from build123d import *

# Parameters (mm, degrees)
F1_DEPTH  = 35
F0_R      = 7.6
F2_DEPTH  = 35
F3_R      = 2.15
F4_DEPTH  = 35.001
F5_R      = 3.65
F5_R_2    = 2.15
F6_DEPTH  = 31
F8_DEPTH  = 20.601
F9_W      = 0.5
F9_H      = 2
F10_DEPTH = 35.0010001
F11_R     = 1.45
F12_DEPTH = 13.851


with BuildPart() as f1:
    # F0 (on Top) → F1 (new body)
    with BuildSketch(Plane.XY):
        with BuildLine():
            ThreePointArc((10, -3.5156791662), (0, -10.6), (-10, -3.5156791662))
            Line((-10, -3.5156791662), (-10, -80.6))
            Line((-10, -80.6), (10, -80.6))
            Line((10, -80.6), (10, -3.5156791662))
        make_face()
    extrude(amount=-F1_DEPTH)

    # F0 (on Top) → F2 (join)
    with BuildSketch(Plane.XY):
        with BuildLine():
            Line((-3.25, 16.6), (-3.25, 10.0894747138))
            ThreePointArc((-3.25, 10.0894747138), (-9.4955609642, 4.7110850104), (-10, -3.5156791662))
            ThreePointArc((-10, -3.5156791662), (0, -10.6), (10, -3.5156791662))
            ThreePointArc((10, -3.5156791662), (9.4955609642, 4.7110850104), (3.25, 10.0894747138))
            Line((3.25, 10.0894747138), (3.25, 16.6))
            Line((3.25, 16.6), (-3.25, 16.6))
        make_face()
        Circle(F0_R, mode=Mode.SUBTRACT)
    extrude(amount=-F2_DEPTH)

    # F3 (on face) → F4 (cut, through all)
    with BuildSketch(Plane.XY):
        with Locations((0, -50.6)):
            Circle(F3_R)
        with Locations((0, -70.6)):
            Circle(F3_R)
    extrude(amount=-F4_DEPTH, mode=Mode.SUBTRACT)

    # F5 (on face) → F6 (cut)
    with BuildSketch(Plane(origin=(0, 0, -35), x_dir=(1, 0, 0), z_dir=(0, 0, -1))):
        with Locations((0, 70.6)):
            Circle(F5_R)
        with Locations((0, 70.6)):
            Circle(F5_R_2, mode=Mode.SUBTRACT)
        with Locations((0, 50.6)):
            Circle(F5_R)
        with Locations((0, 50.6)):
            Circle(F5_R_2, mode=Mode.SUBTRACT)
    extrude(amount=-F6_DEPTH, mode=Mode.SUBTRACT)

    # F7 (on face) → F8 (cut, through all)
    with BuildSketch(Plane.YZ.offset(10)):
        with BuildLine():
            Line((-80.6, -35), (-10.0156791662, -35))
            add(Edge.make_bspline(
                [(-10.0156791662, -35), (-10.0156791662, -5), (-80.6, -5)],
                knots=[0, 0, 0, 1.5707963268, 1.5707963268, 1.5707963268], degree=2, weights=[1, 0.7071067812, 1]))
            Line((-80.6, -5), (-80.6, -35))
        make_face()
    extrude(amount=-F8_DEPTH, mode=Mode.SUBTRACT)

    # F9 (on face) → F10 (cut, through all)
    with BuildSketch(Plane.XY):
        with BuildLine():
            Line((0.5, 16.6), (0, 16.6))
            Line((0, 16.6), (0, 7.6))
            ThreePointArc((0, 7.6), (0.2501355147, 7.5958825836), (0.5, 7.5835347959))
            Line((0.5, 7.5835347959), (0.5, 16.6))
        make_face()
        with BuildLine():
            Line((0, 0), (0, 7.6))
            ThreePointArc((0, 7.6), (-0.2501355147, 7.5958825836), (-0.5, 7.5835347959))
            Line((-0.5, 7.5835347959), (-0.5, 0))
            Line((-0.5, 0), (0, 0))
        make_face()
        with Locations((-0.25, 17.6)):
            Rectangle(F9_W, F9_H)
        with Locations((0.25, 17.6)):
            Rectangle(F9_W, F9_H)
        with BuildLine():
            ThreePointArc((0.5, 7.5835347959), (0.2501355147, 7.5958825836), (0, 7.6))
            Line((0, 7.6), (0, 0))
            Line((0, 0), (0.5, 0))
            Line((0.5, 0), (0.5, 7.5835347959))
        make_face()
        with BuildLine():
            Line((0, 7.6), (0, 16.6))
            Line((0, 16.6), (-0.5, 16.6))
            Line((-0.5, 16.6), (-0.5, 7.5835347959))
            ThreePointArc((-0.5, 7.5835347959), (-0.2501355147, 7.5958825836), (0, 7.6))
        make_face()
    extrude(amount=-F10_DEPTH, mode=Mode.SUBTRACT)

    # F11 (on face) → F12 (cut, through all)
    with BuildSketch(Plane.YZ.offset(3.25)):
        with Locations((13.6, -8.75)):
            Circle(F11_R)
        with Locations((13.6, -26.25)):
            Circle(F11_R)
    extrude(amount=-F12_DEPTH, mode=Mode.SUBTRACT)


solid = f1.part
Here's how the part is built. I have some questions about the finished solid (model axes, mm). A direction names the side the tool comes from. Give positions to 0.01 mm unless a question says otherwise; leave off trailing zeros. Write each loop counter-clockwise with the first axis right and the second up, starting at its lowest first coordinate (ties: lowest second). Pieces come first, ordered by that corner, then holes. Notation, with made-up numbers: (64.25, 84) -> (69.25, 84) arc R15 ccw to (69.25, 111) -> close; hole circle Ø10 at (87, 45.25). An arc over 180 degrees is marked (long way). Use one line per item in the form item = value. Start each with the question number.
1. If I drill on L1, parallel to Y at x = 0, z = -2.1; L2, parallel to Z at x = -2, y = 13.6; L3, parallel to X at y = -70.6, z = -2.1, over which ranges is the centre line in solid material (lowest first)?
2. Thinking about a two-plate mould opening in Y: for faces 1 (the face through (-0.791, -47.037, -5.832)), 2 (the face through (-10, -24, -9)), 3 (the face through (2, 16.6, -17)), which applies, +Y half, -Y half, draft (parallel to the pull), parting line (faces both ways), or undercut?
3. Imagine slicing it at A-A on y = 13.6. List the corners of the cut face in (x, z) for me.
4. Imagine slicing it at B-B on z = -26.25. State how many separate pieces and enclosed holes the cut face has, plus the area to 3 significant figures.
5. Will these pins go through, and if not, where does the flat tip stop? pin 1 Ø4 at (y, z) = (13.6, -26.25) entering from +X; pin 2 Ø3 at (x, y) = (5, -52) entering from -Z; pin 3 Ø2 at (y, z) = (-1, -24) entering from -X; pin 4 Ø1.5 at (x, z) = (-3, -26.5) entering from -Y.
6. On a 3-axis mill with a long thin cutter (end or side, diameter ignored), from which of +Z, -Z, +X, -X, +Y, -Y can I reach the whole of each face in a straight line? I mean faces 4 (the face through (10, -25, -9)), 5 (the face through (2, -69, -4)), 6 (the face through (3.25, 13, -17)). Say none if no direction works.
Entries:
q1.L1 = -80.6 to -72.75, -68.45 to -52.75, -48.45 to -7.6
q1.L2 = -35 to -27.7, -24.8 to -10.2, -7.3 to 0
q1.L3 = -10 to -2.15, 2.15 to 10
q2.face_1 = undercut
q2.face_2 = draft
q2.face_3 = +Y half
q3.outline = (-3.25, -35) -> (-0.5, -35) -> (-0.5, -27.7) -> (-3.25, -27.7) -> close; (-3.25, -24.8) -> (-0.5, -24.8) -> (-0.5, -10.2) -> (-3.25, -10.2) -> close; (-3.25, -7.3) -> (-0.5, -7.3) -> (-0.5, 0) -> (-3.25, 0) -> close; (0.5, -35) -> (3.25, -35) -> (3.25, -27.7) -> (0.5, -27.7) -> close; (0.5, -24.8) -> (3.25, -24.8) -> (3.25, -10.2) -> (0.5, -10.2) -> close; (0.5, -7.3) -> (3.25, -7.3) -> (3.25, 0) -> (0.5, 0) -> close
q4.separate_pieces = 3
q4.enclosed_holes = 0
q4.area = 275 mm²
q5.pin_1 = 3.25
q5.pin_2 = -7.86
q5.pin_3 = -10.6
q5.pin_4 = -13.45
q6.face_4 = +Z, -Z, +X, -Y
q6.face_5 = -Z
q6.face_6 = +Z, -Z, +X, +Y
